Drawing for the job (mm, zero at the part's lowest x, y, z). A direction names the side the tool comes from. Coordinates: 2 decimals unless noted, no trailing zeros. Order: outer loops, then holes, each group sorted by start corner. A loop starts at its lowest first (then second) coordinate and runs counter-clockwise, first axis right, second up. Notation, with made-up numbers: (64.25, 39) -> (114.25, 39) arc R32 ccw to (114.25, 66) -> close; hole circle Ø1 at (66, 64.5). An arc over 180 degrees is marked (long way). Write each question's results on one line, items separated by ' | '.
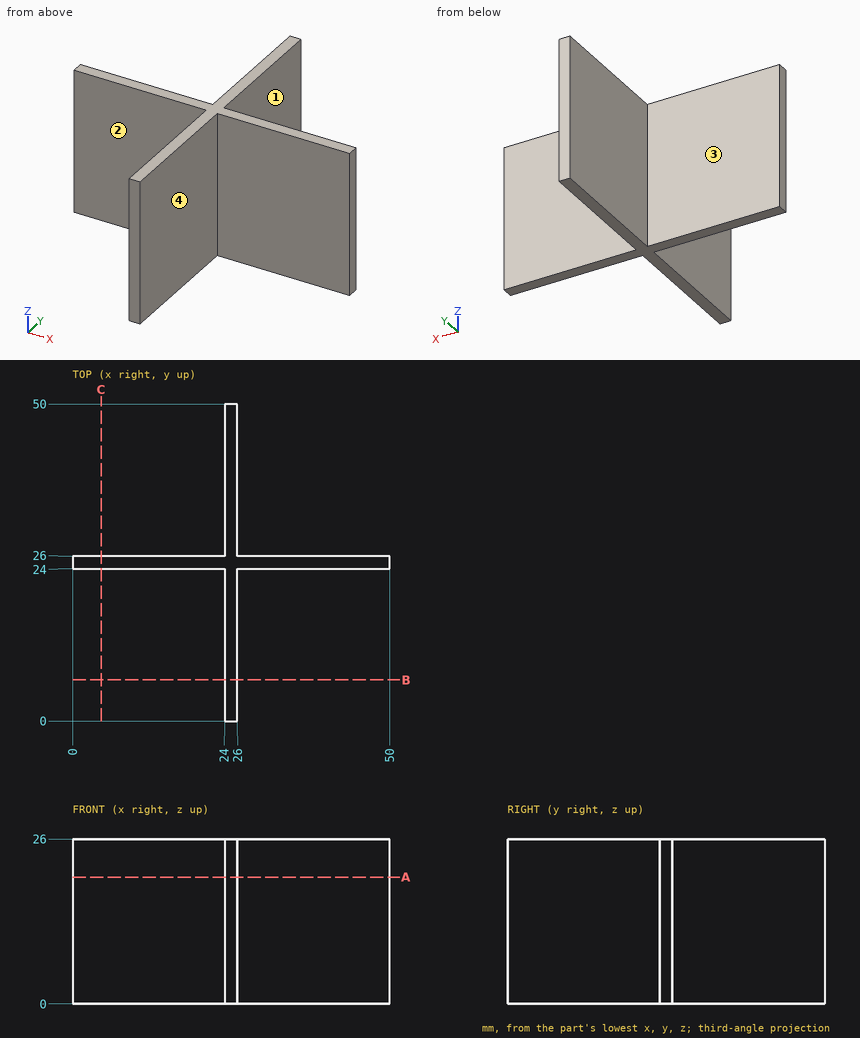
Item 1: Tool access for the marked faces 1, 2, 3 and 4: list every direction of +Z, -Z, +X, -X, +Y, -Y with a clear straight run to the whole face (end or side of a thin tool).
Answer:
face 1: +Z, -Z, +X, +Y | face 2: +Z, -Z, -X, -Y | face 3: +Z, -Z, -X, +Y | face 4: +Z, -Z, +X, -Y
Item 2: Slice it at B-B, the plane y = 6.5. List the corners of the cut face in (x, z), and give its area (3 significant figures).
Answer:
outline: (24, 0) -> (26, 0) -> (26, 26) -> (24, 26) -> close | area: 52.0 mm^2
Item 3: Slice it at A-A, the plane z = 20. List the corners of the cut face in (x, y), and give its area (3 significant figures).
Answer:
outline: (0, 24) -> (24, 24) -> (24, 0) -> (26, 0) -> (26, 24) -> (50, 24) -> (50, 26) -> (26, 26) -> (26, 50) -> (24, 50) -> (24, 26) -> (0, 26) -> close | area: 196 mm^2
Item 4: Drill centre line: line 1 (Y direction, x = 3, z = 6.25). Where is it in solid material? Low to high. Write a range as from..to.
Answer:
line 1: y = 24..26
Item 5: Pin check, flat tips, straight feed: pin 1 (1 mm diameter, centred on x = 43.5, z = 10.5, fed in from -Y); pin 2 (1.5 mm diameter, centred on x = 15, z = 23, fed in from +Y); pin 3 (3 mm diameter, centred on x = 21, y = 39, fed in from +Z); pin 4 (1 mm diameter, centred on y = 12.5, z = 22, fed in from -X). Stop position of each tip, or through.
Answer:
pin 1: stops at y = 24 | pin 2: stops at y = 26 | pin 3: passes through | pin 4: stops at x = 24
